```python
from build123d import *

# Parameters (mm, degrees)
PAD_DEPTH       = 12
POCKET_DEPTH    = 1
FILLET_R        = 20
FILLET001_R     = 20
FILLET002_R     = 20
POCKET001_DEPTH = 5


with BuildPart() as part:
    # Sketch001 → Pad (new body)
    with BuildSketch(Plane.XZ):
        Polygon((-20, -20), (-20, 110), (136.232082, 151.86226), (292.061476, 580), (480, 511.595971), (480, -20), align=None)
    extrude(amount=-PAD_DEPTH)

    # Sketch002 (on Face7 of Pad) → Pocket (cut)
    with BuildSketch(Plane.XZ):
        Polygon((465, -5), (465, 501.092858), (301.026563, 560.774309), (147.656805, 139.394363), (-5, 98.490095), (-5, -5), align=None)
    extrude(amount=POCKET_DEPTH, mode=Mode.SUBTRACT)

    # Fillet
    fillet_edges = [part.edges().sort_by_distance(p)[0] for p in [
        (-20, 6, 110),
    ]]
    fillet(fillet_edges, radius=FILLET_R)

    # Fillet001
    fillet001_edges = [part.edges().sort_by_distance(p)[0] for p in [
        (136.232082, 6, 151.86226),
    ]]
    fillet(fillet001_edges, radius=FILLET001_R)

    # Fillet002
    fillet002_edges = [part.edges().sort_by_distance(p)[0] for p in [
        (292.061476, 6, 580),
    ]]
    fillet(fillet002_edges, radius=FILLET002_R)

    # Sketch003 (on Face7 of Pocket) → Pocket001 (cut)
    with BuildSketch(Plane.XZ):
        Polygon((328.82826, 540.013541), (156.108087, 65.468767), (151.409624, 67.178868), (324.129797, 541.723641), align=None)
    extrude(amount=-POCKET001_DEPTH, mode=Mode.SUBTRACT)


solid = part.part
```
CAD build for the part. Positions are in the model's coordinates, mm. A direction names the side the tool comes from. Round coordinates to 2 decimals unless told otherwise and drop trailing zeros. Order: outer loops, then holes, each group sorted by start corner. A loop starts at its lowest first (then second) coordinate and runs counter-clockwise, first axis right, second up.
Item 1: Saw through at D-D on x = 74. Write the cut outline in (y, z).
Item 2: Probe line 1 along Y through (x, z) = (155.5, 71); line 2 along X through (y, z) = (1, 268); line 3 along Z through (x, y) = (382, 7). List the from-to ranges inside material, lowest first.
Item 3: Saw through at C-C on x = 206. Write the cut outline in (y, z).
Item 4: Tool access for faces 1 (the face through (394.24, 5.92, 542.81)), 2 (the face through (236.56, 2.46, 301.13)): list every direction of +Z, -Z, +X, -X, +Y, -Y with a clear straight run to the whole face (end or side of a thin tool).
Item 5: Mould opens along X. For faces 3 (the face through (241, 5, 305)), 4 (the face through (233, 6, -20)), 5 (the face through (-15.98, 6.08, 106.68)), 6 (the face through (295.364, 6.084, 572.398)) say: pulls with the +X half, pulls with the -X half, needs draft (parallel to the pull), parting line crosses it, or undercut.
Item 6: Saw through at B-B on z = 396. Write the cut outline in (x, y).
Item 7: Saw through at A-A on y = 8. Write the cut outline in (x, z), then the cut area to 3 significant figures.
Item 8: Pin check, flat tips, straight feed: pin 1 (1 mm diameter, centred on y = 2, z = 436.5, fed in from -X); pin 2 (1 mm diameter, centred on x = 401.5, y = 2, fed in from +Z). Stop position of each tip, or through.
Reported:
1. outline: (0, -20) - (12, -20) - (12, 135.19) - (0, 135.19) - close
2. line 1: y = 5 to 12
2. line 2: x = 178.5 to 224.5, 229.82 to 480
2. line 3: z = -20 to 547.27
3. outline: (0, -20) - (12, -20) - (12, 343.55) - (0, 343.55) - (0, 217.16) - (5, 217.16) - (5, 202.55) - (0, 202.55) - close
4. face 1: +Z, +X, +Y, -Y
4. face 2: -Y
5. face 3: undercut
5. face 4: needs draft
5. face 5: pulls with the -X half
5. face 6: parting line crosses it
6. outline: (225.09, 0) - (271.09, 0) - (271.09, 5) - (276.41, 5) - (276.41, 0) - (480, 0) - (480, 12) - (225.09, 12) - close
7. outline: (-20, -20) - (480, -20) - (480, 511.6) - (310.86, 573.16) arc R20 ccw to (285.22, 561.21) - (139.79, 161.65) arc R20 cw to (126.18, 149.17) - (-5.18, 113.97) arc R20 ccw to (-20, 94.65) - close
7. area: 190,000 mm2
8. pin 1: stops at x = 239.65
8. pin 2: stops at z = 540.35
